```python
from build123d import *

# Parameters (mm, degrees)
F0_W     = 20
F0_H     = 50
F0_R     = 2.5
F1_DEPTH = 20
F2_R     = 0.5
F3_R     = 0.5
F4_R     = 0.5
F5_R     = 0.5


with BuildPart() as f1:
    # F0 (on Top) → F1 (new body)
    with BuildSketch(Plane.XY):
        with Locations((-34.2786995421, 5.5646058172)):
            Rectangle(F0_W, F0_H)
        with Locations((-34.2786995421, -9.4353941828)):
            Circle(F0_R, mode=Mode.SUBTRACT)
        with Locations((-34.2786995421, 20.5646058172)):
            Circle(F0_R, mode=Mode.SUBTRACT)
    extrude(amount=F1_DEPTH)

    # F2
    f2_edges = [f1.edges().sort_by_distance(p)[0] for p in [
        (-36.7787, 20.564606, 20),
    ]]
    fillet(f2_edges, radius=F2_R)

    # F3
    f3_edges = [f1.edges().sort_by_distance(p)[0] for p in [
        (-31.7787, -9.435394, 10),
        (-36.7787, -9.435394, 0),
        (-36.7787, -9.435394, 20),
    ]]
    fillet(f3_edges, radius=F3_R)

    # F4
    f4_edges = [f1.edges().sort_by_distance(p)[0] for p in [
        (-36.7787, 20.564606, 0),
    ]]
    fillet(f4_edges, radius=F4_R)

    # F5
    f5_edges = [f1.edges().sort_by_distance(p)[0] for p in [
        (-44.2787, -19.435394, 10),
        (-37.2787, 20.564606, 0),
        (-37.2787, -9.435394, 0),
        (-34.2787, 30.564606, 0),
        (-44.2787, 5.564606, 0),
        (-34.2787, -19.435394, 0),
        (-24.2787, 5.564606, 0),
        (-24.2787, 30.564606, 10),
        (-44.2787, 30.564606, 10),
        (-34.2787, 30.564606, 20),
        (-44.2787, 5.564606, 20),
        (-37.2787, -9.435394, 20),
        (-37.2787, 20.564606, 20),
        (-34.2787, -19.435394, 20),
        (-24.2787, 5.564606, 20),
        (-24.2787, -19.435394, 10),
        (-36.7787, -9.435394, 19.5),
        (-36.7787, 20.564606, 19.5),
        (-36.7787, -9.435394, 0.5),
        (-36.7787, 20.564606, 0.5),
    ]]
    fillet(f5_edges, radius=F5_R)


solid = f1.part
```
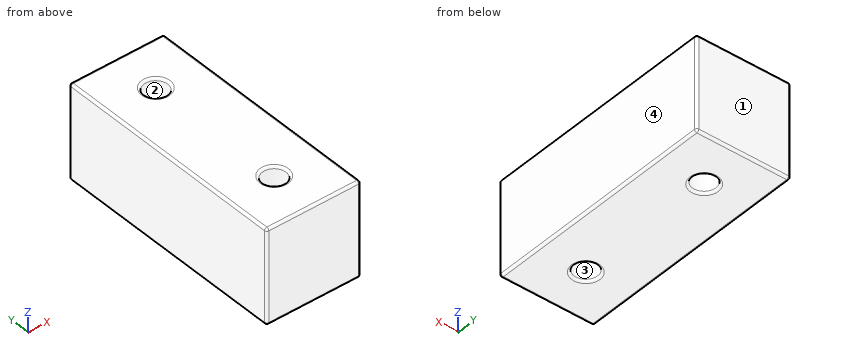
CAD build for the part. Positions are in the model's coordinates, mm. Face numbers are marked on the shaded views. Round coordinates to 2 decimals unless told otherwise and drop trailing zeros. Order: outer loops, then holes, each group sorted by start corner. A loop starts at its lowest first (then second) coordinate and runs counter-clockwise, first axis right, second up. Notation, with made-up numbers: (-7, 19) - (12, 19) arc R12 cw to (12, 33) - close; hole circle Ø6 at (-14.5, -6.5). An arc over 180 degrees is marked (long way). Answer as CSV lines item,"result". Start each with the question number.
1. Saw through at A-A, the plane z = 14. Write the cut outline in (x, y), and give its area (3 significant figures).
2. Pull direction Y, two halves, no side cores. Call the marked faces 1, 2, 3 and 4: +Y half, -Y half, draft (parallel to the pull), parting line (faces both ways), or undercut.
3. Drill centre lines: L1, parallel to Y at x = -34.25, z = 19; L2, parallel to X at y = 20.5, z = 1.75; L3, parallel to Y at x = -36.5, z = 19. Where is each one in solid material? Low to high. Write a range as [from, to].
Model answer:
1,outline,"(-44.28, -18.94) arc R0.5 ccw to (-43.78, -19.44) - (-24.78, -19.44) arc R0.5 ccw to (-24.28, -18.94) - (-24.28, 30.06) arc R0.5 ccw to (-24.78, 30.56) - (-43.78, 30.56) arc R0.5 ccw to (-44.28, 30.06) - close; hole circle Ø5 at (-34.28, -9.44); hole circle Ø5 at (-34.28, 20.56)"
1,area,"961 mm²"
2,face 1,"+Y half"
2,face 2,"undercut"
2,face 3,"undercut"
2,face 4,"draft"
3,L1,"y = [-19.44, -11.94], [-6.94, 18.06], [23.06, 30.56]"
3,L2,"x = [-44.28, -36.78], [-31.78, -24.28]"
3,L3,"y = [-19.44, -10.58], [-8.29, 19.42], [21.71, 30.56]"
